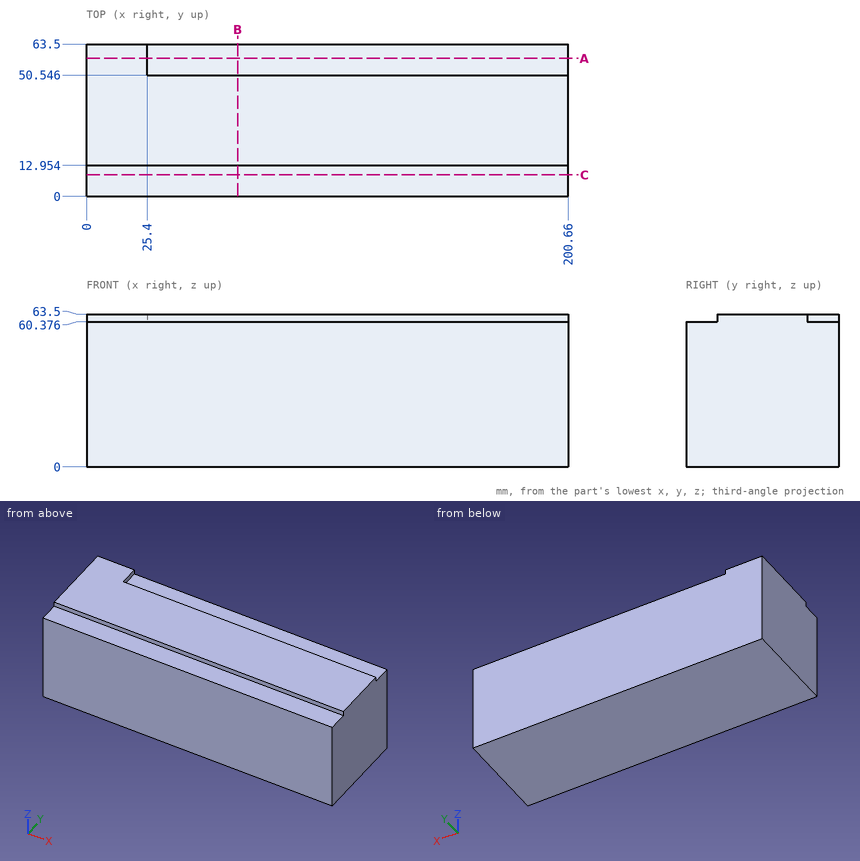
Study the drawing (mm; zero at the part's minimum x, y, z) and answer. Round coordinates to 2 decimals unless told otherwise and drop trailing zeros. Write each loop counter-clockwise with the first axis right and the second up, starting at its lowest first coordinate (ties: lowest second). Pieces come first, ordered by that corner, then holes.
Q1. Find section A-A on y = 57.5. Determine the outline of the cut face in (x, z).
Values:
outline: (0, 0) - (200.66, 0) - (200.66, 60.38) - (25.4, 60.38) - (25.4, 63.5) - (0, 63.5) - close
Q2. A straight line is drawn through the part: line 1 (Z direction, x = 30.5, y = 52.5). Find the intervals that lie inside material, in ascending order.
Values:
line 1: z = 0 to 60.38
Q3. Flat-ended cylindrical pins translate along their axes: P1, Ø1.6, axis at x = 83, z = 62.5, coming from the +Y side; P2, Ø1.6, axis at y = 55, z = 62, coming from the +X side; P3, Ø1.6, axis at x = 89, z = 61.5, coming from the -Y side. Find the tip coordinate at first contact, or state that the pin passes through.
Values:
P1: stops at y = 50.55
P2: stops at x = 25.4
P3: stops at y = 12.95
Q4. Find section B-B on x = 63. Determine the outline of the cut face in (y, z).
Values:
outline: (0, 0) - (63.5, 0) - (63.5, 60.38) - (50.55, 60.38) - (50.55, 63.5) - (12.95, 63.5) - (12.95, 60.38) - (0, 60.38) - close
Q5. Find section C-C on y = 9. Determine the outline of the cut face in (x, z).
Values:
outline: (0, 0) - (200.66, 0) - (200.66, 60.38) - (0, 60.38) - close
